Part model, mm, in its own coordinate system. A direction names the side the tool comes from. Give positions to 0.01 mm unless a question says otherwise; leave off trailing zeros. Loops run counter-clockwise (first coordinate to the right, second up) from the corner with the lowest first, then second, coordinate; pieces in that order, holes last. Notation, with made-up numbers: M -35,-31.75 L -1,-31.75 A25 cw -1,-16.75 Z; hole C 53,85.25 d9. An arc over 180 degrees is marked long. Answer in a Markdown table with one row per item.
from build123d import *

# Parameters (mm, degrees)
CHAMFER1_SIZE = 1
CHAMFER2_SIZE = 0.5


with BuildPart() as part:
    # Sketch1 → Revolve1 (revolve)
    with BuildSketch(Plane(origin=(0, 0, 0), x_dir=(0, 0, -1), z_dir=(1, 0, 0)), mode=Mode.PRIVATE) as revolve1_sk:
        Polygon((22, 0), (22, 2.0828), (0, 2.0828), (0, 3.5), (-40.879, 3.5), (-40.879, 0), align=None)
    revolve(revolve1_sk.sketch.rotate(Axis((0, 0, 0), (0, 0, -1)), 90), axis=Axis((0, 0, 0), (0, 0, -1)))  # turned: the seam where the file's is

    # Chamfer1
    chamfer1_edges = [part.edges().sort_by_distance(p)[0] for p in [
        (-2.0828, 0, -22),
    ]]
    chamfer(chamfer1_edges, length=CHAMFER1_SIZE)

    # Chamfer2
    chamfer2_edges = [part.edges().sort_by_distance(p)[0] for p in [
        (-3.5, 0, 40.879),
    ]]
    chamfer(chamfer2_edges, length=CHAMFER2_SIZE)


solid = part.part
(1) Saw through at C-C (z = 21). Write the cut outline in (x, y), plus the area to 3 significant figures.
Recorded:
| item | result |
|---|---|
| outline | C 0,0 d7 |
| area | 38.5 mm^2 |
(2) Drill centre lines: line 1 along Z through (x, y) = (-2, -2.25); line 2 along X through (y, z) = (3, 12); line 3 along Y through (x, z) = (-1.5, -17). Where is each one in solid material? Low to high.
Recorded:
| item | result |
|---|---|
| line 1 | z = 0 to 40.87 |
| line 2 | x = -1.8 to 1.8 |
| line 3 | y = -1.45 to 1.45 |
(3) Saw through at A-A (x = 0). Write the cut outline in (y, z).
Recorded:
| item | result |
|---|---|
| outline | M -3.5,0 L -2.08,0 L -2.08,-21 L -1.08,-22 L 1.08,-22 L 2.08,-21 L 2.08,0 L 3.5,0 L 3.5,40.38 L 3,40.88 L -3,40.88 L -3.5,40.38 Z |
(4) Pin check, flat tips, straight feed: pin 1 Ø1 at (y, z) = (-1, -14.5) entering from +X; pin 2 Ø1.5 at (x, y) = (-1, 2.5) entering from -Z; pin 3 Ø2 at (x, y) = (-1, 1.5) entering from -Z; pin 4 Ø3 at (x, y) = (-1, -2.5) entering from -Z. Stop position of each tip, or through.
Recorded:
| item | result |
|---|---|
| pin 1 | stops at x = 2.02 |
| pin 2 | stops at z = -21.14 |
| pin 3 | stops at z = -22 |
| pin 4 | stops at z = -21.89 |
(5) Which spindle directions (+Z, -Z, +X, -X, +Y, -Y) get a long thin tool onto all of the face, cutting with end or side? Do faces 1 (the face through (-2, 2, 0)), 2 (the face through (1.615, 3.105, 20.472)). Say none if no direction does.
Recorded:
| item | result |
|---|---|
| face 1 | -Z |
| face 2 | +Z, -Z |
